Source: CAD feature listing. Evaluate the final solid. Frame: model axes, mm. Face numbers are marked on the shaded views. A direction names the side the tool comes from. Coordinates: 2 decimals unless noted, no trailing zeros. Order: outer loops, then holes, each group sorted by start corner. A loop starts at its lowest first (then second) coordinate and runs counter-clockwise, first axis right, second up.
```python
from build123d import *

# Parameters (mm, degrees)
BOSS_EXTRUDE2_DEPTH      = 25
BOSS_EXTRUDE2_DEPTH_BACK = 25
SKETCH1_R                = 9
SKETCH2_R                = 7.5
BOSS_EXTRUDE3_DEPTH      = 15
FILLET2_R                = 1
CUT_EXTRUDE1_DEPTH       = 42.976183724
CUT_EXTRUDE1_DEPTH_BACK  = 42.976183724
SKETCH3_R                = 3


with BuildPart() as part:
    # Sketch1 → Boss-Extrude2 (new, two sides: drawn at the far end of the back side and taken through both)
    with BuildSketch(Plane(origin=(0, 0, 0), x_dir=(0, 0, -1), z_dir=(1, 0, 0)).offset(-BOSS_EXTRUDE2_DEPTH_BACK)):
        Circle(SKETCH1_R)
    extrude(amount=BOSS_EXTRUDE2_DEPTH + BOSS_EXTRUDE2_DEPTH_BACK)

    # Sketch2 → Boss-Extrude3 (add)
    with BuildSketch(Plane(origin=(25, 0, 0), x_dir=(0, 0, -1), z_dir=(1, 0, 0))):
        Circle(SKETCH2_R)
    boss_extrude3 = extrude(amount=BOSS_EXTRUDE3_DEPTH)

    # Mirror1: Boss-Extrude3 across plane
    add(boss_extrude3.mirror(Plane(origin=(0, 0, 0), x_dir=(0, 0, 1), z_dir=(1, 0, 0))))

    # Fillet2
    fillet2_edges = [part.edges().sort_by_distance(p)[0] for p in [
        (-40, 0, 7.5),
        (40, 0, 7.5),
    ]]
    fillet(fillet2_edges, radius=FILLET2_R)

    # Sketch3 → Cut-Extrude1 (cut, two sides: drawn at the far end of the back side and taken through both)
    with BuildSketch(Plane.XY.offset(-CUT_EXTRUDE1_DEPTH_BACK)):
        Circle(SKETCH3_R)
    extrude(amount=CUT_EXTRUDE1_DEPTH + CUT_EXTRUDE1_DEPTH_BACK, mode=Mode.SUBTRACT)


solid = part.part
```
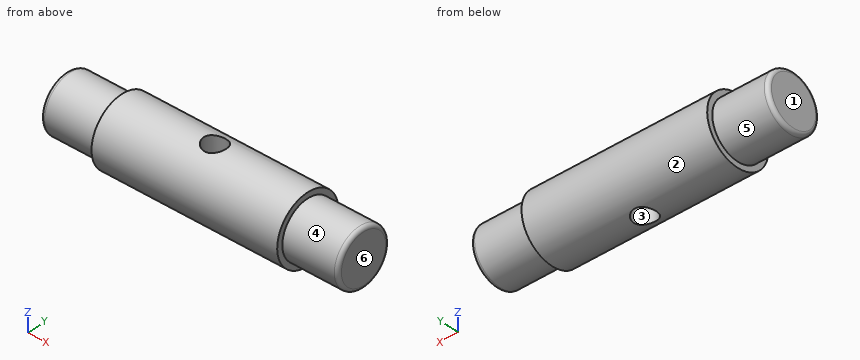
1. Section query B-B on y = 0. Return loops of the section in (x, z).
Findings:
outline: (-40, -6.5) arc R1 ccw to (-39, -7.5) - (-25, -7.5) - (-25, -9) - (-3, -9) - (-3, 9) - (-25, 9) - (-25, 7.5) - (-39, 7.5) arc R1 ccw to (-40, 6.5) - close; (3, -9) - (25, -9) - (25, -7.5) - (39, -7.5) arc R1 ccw to (40, -6.5) - (40, 6.5) arc R1 ccw to (39, 7.5) - (25, 7.5) - (25, 9) - (3, 9) - close
2. Section query A-A on z = 0. Return loops of the section in (x, y), plus the area to 3 significant figures.
Findings:
outline: (-40, -6.5) arc R1 ccw to (-39, -7.5) - (-25, -7.5) - (-25, -9) - (25, -9) - (25, -7.5) - (39, -7.5) arc R1 ccw to (40, -6.5) - (40, 6.5) arc R1 ccw to (39, 7.5) - (25, 7.5) - (25, 9) - (-25, 9) - (-25, 7.5) - (-39, 7.5) arc R1 ccw to (-40, 6.5) - close; hole circle Ø6 at (0, 0)
area: 1,320 mm2
3. Ray query, line 1 (X direction, y = 0, z = -1.75); line 2 (X direction, y = -7, z = -5.5); line 3 (Y direction, x = 0, z = 1). Return the intervals inside material, ascending.
Findings:
line 1: x = -40 to -3, 3 to 40
line 2: x = -25 to 25
line 3: y = -8.94 to -3, 3 to 8.94
4. Pin query (flat end, axial travel): P1, Ø4, axis at x = 4.5, z = 2.5, coming from the +Y side; P2, Ø2, axis at x = 27.5, z = -7, coming from the -Y side; P3, Ø6, axis at x = -27.5, z = -5.5, coming from the -Y side. Return the tip coordinate at first contact, or that it passes through.
Findings:
P1: stops at y = 8.99
P2: stops at y = -4.5
P3: stops at y = -8.14
5. Section query D-D on x = 0. Return loops of the section in (y, z).
Findings:
outline: (-3, -8.49) - (-3, 8.49) arc R9 ccw to start; (3, -8.49) arc R9 ccw to (3, 8.49) - close
6. Draft query along Y for the marked faces 1, 2 and 3. Return one class per face: released by +Y, released by -Y, zero draft, split by the parting line, or undercut.
Findings:
face 1: zero draft
face 2: split by the parting line
face 3: undercut
7. Access query for the marked faces 4, 5 and 6. Directions: +Z, -Z, +X, -X, +Y, -Y. A direction counts if a zero-diameter tool reaches every point of the face in a straight line with its end or side. Return the directions, or none.
Findings:
face 4: +X
face 5: -X
face 6: +Z, -Z, +X, +Y, -Y
8. Section query C-C on x = 12. Return loops of the section in (y, z).
Findings:
outline: circle Ø18 at (0, 0)
